CAD build for the part. Positions are in the model's coordinates, mm. Coordinates: 2 decimals unless noted, no trailing zeros. Order: outer loops, then holes, each group sorted by start corner. A loop starts at its lowest first (then second) coordinate and runs counter-clockwise, first axis right, second up. Notation, with made-up numbers: (71.25, 53.5) - (97.25, 53.5) arc R14 cw to (97.25, 73.5) - close; hole circle Ø5 at (88.5, 60.25). An arc over 180 degrees is marked (long way). Write each question's results on one line, items separated by ' | '. Start each with the question number.
Q1. Band-saw the part on D-D, the plane x = -95. Write the cut outline in (y, z), then the cut area to 3 significant figures.
Q2. Band-saw the part on C-C, the plane y = -22. Write the cut outline in (x, z).
Q3. Band-saw the part on A-A, the plane x = 88.5. Write the cut outline in (y, z), then the cut area to 3 significant figures.
Q4. Band-saw the part on B-B, the plane z = 18. Count the separate pieces of the cut face and the enclosed holes in it, then the cut area to 3 significant figures.
Q5. Pin check, flat tips, straight feed: P1, Ø4, axis at y = 22.5, z = 34, coming from the -X side; P2, Ø2, axis at y = 5, z = 2.5, coming from the +X side; P3, Ø8, axis at y = 15, z = 19.5, coming from the +X side. Stop position of each tip, or through.
Q6. Wall check: probe 1 along X at (y, z) = (-19.5, 27); probe 2 along Z at (x, y) = (-155, -5.5); probe 3 along Z at (x, y) = (-113, -24). Give the ranges that are in metal, low to high.
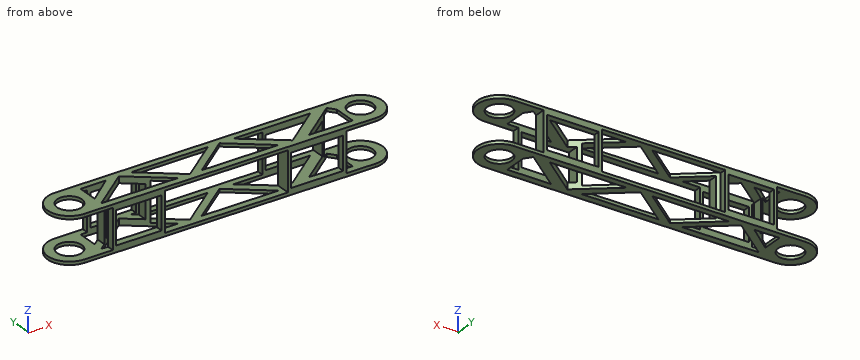
```python
from build123d import *

# Parameters (mm, degrees)
CROQUIS1_R              = 15.25
SALIENTE_EXTRUIR1_DEPTH = 57
CROQUIS2_W              = 70
CROQUIS2_H              = 44
CROQUIS2_W_2            = 152.323993802
CORTAR_EXTRUIR1_DEPTH   = 40
CORTAR_EXTRUIR3_DEPTH   = 75
CROQUIS4_R              = 15.25
CORTAR_EXTRUIR4_DEPTH   = 2.5
CROQUIS5_R              = 15.25
CORTAR_EXTRUIR5_DEPTH   = 2.5
CROQUIS6_R              = 15.083558861
CORTAR_EXTRUIR6_DEPTH   = 2.5
CROQUIS7_R              = 15.25
CORTAR_EXTRUIR7_DEPTH   = 2.5
CROQUIS8_W              = 152.323993802
CROQUIS8_H              = 54
CORTAR_EXTRUIR8_DEPTH   = 2.5
CROQUIS9_W              = 152.323993802
CROQUIS9_H              = 54
CORTAR_EXTRUIR9_DEPTH   = 2.5
CROQUIS10_W             = 56.441876841
CROQUIS10_H             = 41
CORTAR_EXTRUIR10_DEPTH  = 70
CROQUIS11_W             = 64.296395464
CROQUIS11_H             = 41
CORTAR_EXTRUIR11_DEPTH  = 70
CORTAR_EXTRUIR12_DEPTH  = 78


with BuildPart() as part:
    # Croquis1 → Saliente-Extruir1 (new body)
    with BuildSketch(Plane.XY):
        with BuildLine():
            Line((-180, -35), (180, -35))
            ThreePointArc((180, -35), (215, 0), (180, 35))
            Line((180, 35), (-180, 35))
            ThreePointArc((-180, 35), (-215, 0), (-180, -35))
        make_face()
        with Locations((-180, 0)):
            Circle(CROQUIS1_R, mode=Mode.SUBTRACT)
        with Locations((180, 0)):
            Circle(CROQUIS1_R, mode=Mode.SUBTRACT)
    extrude(amount=SALIENTE_EXTRUIR1_DEPTH)

    # Croquis2 → Cortar-Extruir1 (cut, symmetric)
    with BuildSketch(Plane(origin=(0, 0, 0), x_dir=(1, 0, 0), z_dir=(0, 1, 0))):
        with Locations((-180, -28.5)):
            Rectangle(CROQUIS2_W, CROQUIS2_H)
        with Locations((179.062266107, -28.5)):
            Rectangle(CROQUIS2_W, CROQUIS2_H)
        with Locations((-4.396126258, -28.5)):
            Rectangle(CROQUIS2_W_2, CROQUIS2_H)
    extrude(amount=CORTAR_EXTRUIR1_DEPTH, both=True, mode=Mode.SUBTRACT)

    # Croquis3 → Cortar-Extruir3 (cut, symmetric)
    with BuildSketch(Plane.XY):
        with BuildLine():
            Line((-180, -35), (180, -35))
            ThreePointArc((180, -35), (215, 0), (180, 35))
            Line((180, 35), (-180, 35))
            ThreePointArc((-180, 35), (-215, 0), (-180, -35))
        make_face()
        with BuildLine():
            Line((-180, -27), (180, -27))
            ThreePointArc((180, -27), (207, 0), (180, 27))
            Line((180, 27), (-180, 27))
            ThreePointArc((-180, 27), (-207, 0), (-180, -27))
        make_face(mode=Mode.SUBTRACT)
    extrude(amount=CORTAR_EXTRUIR3_DEPTH, both=True, mode=Mode.SUBTRACT)

    # Croquis4 → Cortar-Extruir4 (cut)
    with BuildSketch(Plane.XY.offset(6.5)):
        with BuildLine():
            Line((-145, 27), (-180, 27))
            ThreePointArc((-180, 27), (-207, 0), (-180, -27))
            Line((-180, -27), (-145, -27))
            Line((-145, -27), (-145, 27))
        make_face()
        with Locations((-180, 0)):
            Circle(CROQUIS4_R, mode=Mode.SUBTRACT)
    extrude(amount=-CORTAR_EXTRUIR4_DEPTH, mode=Mode.SUBTRACT)

    # Croquis5 → Cortar-Extruir5 (cut)
    with BuildSketch(Plane(origin=(0, 0, 50.5), x_dir=(-1, 0, 0), z_dir=(0, 0, -1))):
        with BuildLine():
            Line((180, 27), (145, 27))
            Line((145, 27), (145, -27))
            Line((145, -27), (180, -27))
            ThreePointArc((180, -27), (207, 0), (180, 27))
        make_face()
        with Locations((180, 0)):
            Circle(CROQUIS5_R, mode=Mode.SUBTRACT)
    extrude(amount=-CORTAR_EXTRUIR5_DEPTH, mode=Mode.SUBTRACT)

    # Croquis6 → Cortar-Extruir6 (cut)
    with BuildSketch(Plane.XY.offset(6.5)):
        with BuildLine():
            Line((180, 27), (144.062266107, 27))
            Line((144.062266107, 27), (144.062266107, -27))
            Line((144.062266107, -27), (180, -27))
            ThreePointArc((180, -27), (207, 0), (180, 27))
        make_face()
        with Locations((180, 0)):
            Circle(CROQUIS6_R, mode=Mode.SUBTRACT)
    extrude(amount=-CORTAR_EXTRUIR6_DEPTH, mode=Mode.SUBTRACT)

    # Croquis7 → Cortar-Extruir7 (cut)
    with BuildSketch(Plane(origin=(0, 0, 50.5), x_dir=(-1, 0, 0), z_dir=(0, 0, -1))):
        with BuildLine():
            Line((-180, -27), (-144.062266107, -27))
            Line((-144.062266107, -27), (-144.062266107, 27))
            Line((-144.062266107, 27), (-180, 27))
            ThreePointArc((-180, 27), (-207, 0), (-180, -27))
        make_face()
        with Locations((-180, 0)):
            Circle(CROQUIS7_R, mode=Mode.SUBTRACT)
    extrude(amount=-CORTAR_EXTRUIR7_DEPTH, mode=Mode.SUBTRACT)

    # Croquis8 → Cortar-Extruir8 (cut)
    with BuildSketch(Plane(origin=(0, 0, 50.5), x_dir=(-1, 0, 0), z_dir=(0, 0, -1))):
        with Locations((4.396126258, 0)):
            Rectangle(CROQUIS8_W, CROQUIS8_H)
    extrude(amount=-CORTAR_EXTRUIR8_DEPTH, mode=Mode.SUBTRACT)

    # Croquis9 → Cortar-Extruir9 (cut)
    with BuildSketch(Plane.XY.offset(6.5)):
        with Locations((-4.396126258, 0)):
            Rectangle(CROQUIS9_W, CROQUIS9_H)
    extrude(amount=-CORTAR_EXTRUIR9_DEPTH, mode=Mode.SUBTRACT)

    # Croquis10 → Cortar-Extruir10 (cut)
    with BuildSketch(Plane(origin=(0, 27, 0), x_dir=(1, 0, 0), z_dir=(0, 1, 0))):
        with Locations((-112.779061579, -28.5)):
            Rectangle(CROQUIS10_W, CROQUIS10_H)
    extrude(amount=-CORTAR_EXTRUIR10_DEPTH, mode=Mode.SUBTRACT)

    # Croquis11 → Cortar-Extruir11 (cut)
    with BuildSketch(Plane(origin=(0, 27, 0), x_dir=(1, 0, 0), z_dir=(0, 1, 0))):
        with Locations((107.914068375, -28.5)):
            Rectangle(CROQUIS11_W, CROQUIS11_H)
    extrude(amount=-CORTAR_EXTRUIR11_DEPTH, mode=Mode.SUBTRACT)

    # Croquis12 → Cortar-Extruir12 (cut)
    with BuildSketch(Plane.XY.offset(57)):
        Polygon((-153.246746746, -18.260795107), (-105.980425778, 18.9839027), (-58.446911177, -18.260795107), align=None)
        Polygon((-153.246746746, 18.9839027), (-122.113012552, 18.9839027), (-153.246746746, -6.441367348), align=None)
        Polygon((157.831126984, 10.304103568), (157.831126984, -18.260795107), (103.74320228, -18.260795107), (150.988634974, 18.9839027), align=None)
        Polygon((-90.712084725, 18.9839027), (-43.46665203, -18.260795107), (4.066862571, 18.9839027), align=None)
        Polygon((-29.062556696, -18.260795107), (18.470957905, 18.9839027), (66.004472506, -18.260795107), align=None)
        Polygon((35.755872305, 18.9839027), (83.577468813, -18.260795107), (130.822901507, 18.9839027), align=None)
    extrude(amount=-CORTAR_EXTRUIR12_DEPTH, mode=Mode.SUBTRACT)


solid = part.part
```
Results below:
1) outline: (-27, 0) - (-18.26, 0) - (-18.26, 8) - (-27, 8) - close; (-27, 49) - (-18.26, 49) - (-18.26, 57) - (-27, 57) - close; (10.38, 0) - (27, 0) - (27, 8) - (10.38, 8) - close; (10.38, 49) - (27, 49) - (27, 57) - (10.38, 57) - close | area: 406 mm²
2) outline: (-195.65, 0) - (195.65, 0) - (195.65, 4) - (144.06, 4) - (144.06, 53) - (195.65, 53) - (195.65, 57) - (-195.65, 57) - (-195.65, 53) - (-145, 53) - (-145, 4) - (-195.65, 4) - close; hole (-141, 8) - (-84.56, 8) - (-84.56, 49) - (-141, 49) - close; hole (-80.56, 4) - (71.77, 4) - (71.77, 53) - (-80.56, 53) - close; hole (75.77, 8) - (140.06, 8) - (140.06, 49) - (75.77, 49) - close
3) outline: (-27, 0) - (-14.38, 0) - (-14.38, 8) - (-27, 8) - close; (-27, 49) - (-14.38, 49) - (-14.38, 57) - (-27, 57) - close; (18.98, 0) - (27, 0) - (27, 8) - (18.98, 8) - close; (18.98, 49) - (27, 49) - (27, 57) - (18.98, 57) - close | area: 330 mm²
4) separate pieces: 10 | enclosed holes: 0 | area: 423 mm²
5) P1: stops at x = -145 | P2: stops at x = 206.7 | P3: stops at x = 144.06
6) probe 1: x = -145 to -141, -84.56 to -80.56, 71.77 to 75.77, 140.06 to 144.06 | probe 2: z = 0 to 4, 53 to 57 | probe 3: z = 0 to 8, 49 to 57
